Part model, mm, in its own coordinate system. A direction names the side the tool comes from. Coordinates: 2 decimals unless noted, no trailing zeros. Loops run counter-clockwise (first coordinate to the right, second up) from the corner with the lowest first, then second, coordinate; pieces in that order, holes last. Notation, with made-up numbers: (-18.5, -3.5) - (40.5, -3.5) arc R25 ccw to (40.5, 16.5) - close; hole circle Ø10 at (25.25, 59). An arc over 180 degrees is marked (long way). Use a Markdown table: item, result. Add a question column.
1) Band-saw the part on C-C (z = 4.5). Give the cut face in (x, y), plus the area to 3 significant figures.
2) Band-saw the part on A-A (y = -2.5). Give the cut face in (x, z).
3) Probe probe 1 along X at (y, z) = (-4.75, 6.5); probe 2 along X at (y, z) = (-4.75, 10); probe 3 along Z at (x, y) = (4, -1). List the from-to ranges inside material, lowest first. Write a range as [from, to].
4) Tool access for faces 4 (the face through (0, -6.35, -4)), 5 (the face through (-5.245, -3.131, 5.361)): list every direction of +Z, -Z, +X, -X, +Y, -Y with a clear straight run to the whole face (end or side of a thin tool).
5) Pull direction Z, two halves, no side cores. Call faces 1 (the face through (0, 0, -4)), 2 (the face through (5.245, -3.131, -5.361)), 3 (the face through (-4.336, -3.131, -19.524)): +Z half, -Z half, draft (parallel to the pull), parting line (faces both ways), or undercut.
6) Drop flat-ended pins along their axis: P1, Ø2, axis at y = -4, z = -14, coming from the -X side; P2, Ø2, axis at y = -2.5, z = 16, coming from the +X side; P3, Ø1.5, axis at x = -10.5, y = -5, coming from the +Z side. Give the stop position or say it passes through.
7) Band-saw the part on D-D (x = -1). Give the cut face in (y, z), plus the area to 3 significant figures.
8) Band-saw the part on B-B (x = -5). Give the cut face in (y, z).
from build123d import *

# Parameters (mm, degrees)
F0_R     = 20
F0_R_2   = 2.0000994159
F1_DEPTH = 6.35


# Not quite as in the source:
# - a length typed as a fraction of an inch, garbled in the dataset ("3 / 203.2 mm" for 3/8 in), is restored


with BuildPart() as f1:
    # F0 (on Front) → F1 (new body)
    with BuildSketch(Plane.XZ):
        Circle(F0_R)
        with BuildLine():
            ThreePointArc((0, 15), (10.6066017178, 10.6066017178), (15, 0))
            ThreePointArc((15, 0), (10.6066017178, -10.6066017178), (0, -15))
            ThreePointArc((0, -15), (-10.6066017178, -10.6066017178), (-15, 0))
            ThreePointArc((-15, 0), (-10.6066017178, 10.6066017178), (0, 15))
        make_face(mode=Mode.SUBTRACT)
        with BuildLine():
            ThreePointArc((0, -7.5), (5.3033008589, -5.3033008589), (7.5, 0))
            ThreePointArc((7.5, 0), (5.3033008589, 5.3033008589), (0, 7.5))
            ThreePointArc((0, 7.5), (-5.3033008589, 5.3033008589), (-7.5, 0))
            ThreePointArc((-7.5, 0), (-5.3033008589, -5.3033008589), (0, -7.5))
        make_face()
        Circle(F0_R_2, mode=Mode.SUBTRACT)
        with BuildLine():
            ThreePointArc((-15, 0), (-10.6066017178, -10.6066017178), (0, -15))
            Line((0, -15), (0, -7.5))
            ThreePointArc((0, -7.5), (-5.3033008589, -5.3033008589), (-7.5, 0))
            Line((-7.5, 0), (-15, 0))
        make_face()
        with BuildLine():
            Line((7.5, 0), (15, 0))
            ThreePointArc((15, 0), (10.6066017178, 10.6066017178), (0, 15))
            Line((0, 15), (0, 7.5))
            ThreePointArc((0, 7.5), (5.3033008589, 5.3033008589), (7.5, 0))
        make_face()
    extrude(amount=F1_DEPTH)


solid = f1.part
Answer block:
| question | item | result |
|---|---|---|
| 1 | outline | (-19.49, -6.35) - (-14.31, -6.35) - (-14.31, 0) - (-19.49, 0) - close; (-6, -6.35) - (19.49, -6.35) - (19.49, 0) - (-6, 0) - close |
| 1 | area | 195 mm2 |
| 2 | outline | circle Ø40 at (0, 0); hole (-15, 0) - (-7.5, 0) arc R7.5 cw to (0, 7.5) - (0, 15) arc R15 ccw to start; hole circle Ø4 at (0, 0); hole (0, -15) arc R15 ccw to (15, 0) - (7.5, 0) arc R7.5 cw to (0, -7.5) - close |
| 3 | probe 1 | [-18.91, -13.52], [-3.74, 18.91] |
| 3 | probe 2 | [-17.32, -11.18], [0, 17.32] |
| 3 | probe 3 | [-19.6, -14.46], [-6.34, 19.6] |
| 4 | face 4 | +Z, -Z, +X, -X, -Y |
| 4 | face 5 | +Y, -Y |
| 5 | face 1 | draft |
| 5 | face 2 | undercut |
| 5 | face 3 | parting line |
| 6 | P1 | x = -15.2 |
| 6 | P2 | x = 13.23 |
| 6 | P3 | z = 17.46 |
| 7 | outline | (-6.35, -19.97) - (0, -19.97) - (0, -1.73) - (-6.35, -1.73) - close; (-6.35, 1.73) - (0, 1.73) - (0, 7.43) - (-6.35, 7.43) - close; (-6.35, 14.97) - (0, 14.97) - (0, 19.97) - (-6.35, 19.97) - close |
| 7 | area | 184 mm2 |
| 8 | outline | (-6.35, -19.36) - (0, -19.36) - (0, 5.59) - (-6.35, 5.59) - close; (-6.35, 14.14) - (0, 14.14) - (0, 19.36) - (-6.35, 19.36) - close |
